Build history of the part. All positions in model axes, mm. Give positions to 0.01 mm unless a question says otherwise; leave off trailing zeros. Loops run counter-clockwise (first coordinate to the right, second up) from the corner with the lowest first, then second, coordinate; pieces in that order, holes last. Notation, with made-up numbers: M 78,48 L 96,48 A17 cw 96,65 Z; hole C -18,53.5 d5. An arc over 180 degrees is marked long. Answer in a Markdown table with one row per item. Add a question column.
```python
from build123d import *

# Parameters (mm, degrees)
SKETCH_1_R      = 1.5
SKETCH_1_R_2    = 1.55
SKETCH_1_R_3    = 1.6
SKETCH_1_R_4    = 1.65
SKETCH_1_R_5    = 1.7
EXTRUDE_1_DEPTH = 3


with BuildPart() as part:
    # 草图1 → 凸台-拉伸1 (new body)
    with BuildSketch(Plane.XY):
        with BuildLine():
            Line((0, 2.5), (17.5, 2.5))
            Line((17.5, 2.5), (22.5, 2.5))
            Line((22.5, 2.5), (22.5, -2.5))
            Line((22.5, -2.5), (17.5, -2.5))
            Line((17.5, -2.5), (0, -2.5))
            ThreePointArc((0, -2.5), (-2.5, 0), (0, 2.5))
        make_face()
        Circle(SKETCH_1_R, mode=Mode.SUBTRACT)
        with Locations((5, 0)):
            Circle(SKETCH_1_R_2, mode=Mode.SUBTRACT)
        with Locations((10, 0)):
            Circle(SKETCH_1_R_3, mode=Mode.SUBTRACT)
        with Locations((15, 0)):
            Circle(SKETCH_1_R_4, mode=Mode.SUBTRACT)
        with Locations((20, 0)):
            Circle(SKETCH_1_R_5, mode=Mode.SUBTRACT)
    extrude(amount=EXTRUDE_1_DEPTH)


solid = part.part
```
(1) Slice it at A-A, the plane x = 15. Give the cut face in (y, z).
(2) Pull direction Y, two halves, no side cores. Call faces 1 (the cylindrical face through (16.574, 0.496, 1.479)), 2 (the flat face through (11, -2.5, 1)), 3 (the flat face through (10, 2, 0)): +Y half, -Y half, draft (parallel to the pull), parting line (faces both ways), or undercut.
(3) Wall check: line 1 (X direction, y = -0.35, z = 2.95); line 2 (X direction, y = -1, z = 0.85); line 3 (Y direction, x = 20, z = 1.85). Give the ranges that are in metal, low to high.
(4) Slice it at B-B, the plane y = 0. Give the cut face in (x, z).
(5) Slice it at D-D, the plane x = 20. Give the cut face in (y, z), then the cut area to 3 significant figures.
(6) Slice it at C-C, the plane z = 2.5. Give the cut face in (x, y).
Solution:
| question | item | result |
|---|---|---|
| 1 | outline | M -2.5,0 L -1.65,0 L -1.65,3 L -2.5,3 Z; M 1.65,0 L 2.5,0 L 2.5,3 L 1.65,3 Z |
| 2 | face 1 | undercut |
| 2 | face 2 | -Y half |
| 2 | face 3 | draft |
| 3 | line 1 | -2.48 to -1.46, 1.46 to 3.49, 6.51 to 8.44, 11.56 to 13.39, 16.61 to 18.34, 21.66 to 22.5 |
| 3 | line 2 | -2.29 to -1.12, 1.12 to 3.82, 6.18 to 8.75, 11.25 to 13.69, 16.31 to 18.63, 21.37 to 22.5 |
| 3 | line 3 | -2.5 to -1.7, 1.7 to 2.5 |
| 4 | outline | M -2.5,0 L -1.5,0 L -1.5,3 L -2.5,3 Z; M 1.5,0 L 3.45,0 L 3.45,3 L 1.5,3 Z; M 6.55,0 L 8.4,0 L 8.4,3 L 6.55,3 Z; M 11.6,0 L 13.35,0 L 13.35,3 L 11.6,3 Z; M 16.65,0 L 18.3,0 L 18.3,3 L 16.65,3 Z; M 21.7,0 L 22.5,0 L 22.5,3 L 21.7,3 Z |
| 5 | outline | M -2.5,0 L -1.7,0 L -1.7,3 L -2.5,3 Z; M 1.7,0 L 2.5,0 L 2.5,3 L 1.7,3 Z |
| 5 | area | 4.80 mm^2 |
| 6 | outline | M 0,-2.5 L 22.5,-2.5 L 22.5,2.5 L 0,2.5 A2.5 ccw Z; hole C 0,0 d3; hole C 5,0 d3.1; hole C 10,0 d3.2; hole C 15,0 d3.3; hole C 20,0 d3.4 |
